Design review of the part shown in the three views and the two pictorial views. Dimensions are in mm from the part's minimum x, y and z. Give positions to 0.01 mm unless a question says otherwise; leave off trailing zeros. Order: outer loops, then holes, each group sorted by start corner. A loop starts at its lowest first (then second) coordinate and runs counter-clockwise, first axis right, second up.
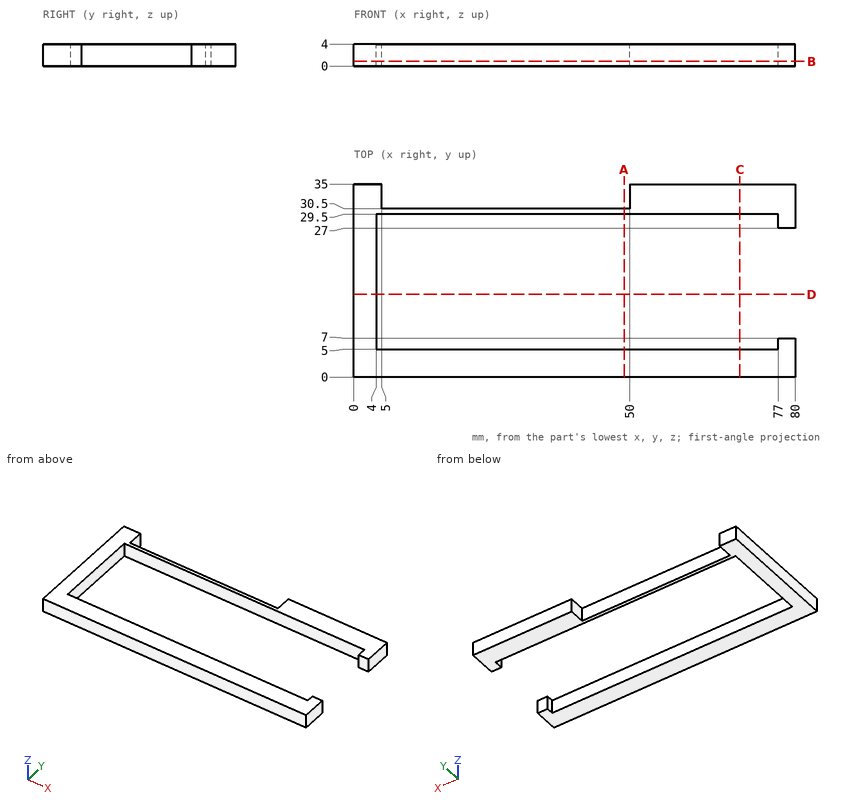
1) We need section A-A on x = 49. Give the boundary of the cut face in (y, z), then the cut area to 3 significant figures.
Answer sheet:
outline: (0, 0) - (5, 0) - (5, 4) - (0, 4) - close; (29.5, 0) - (30.5, 0) - (30.5, 4) - (29.5, 4) - close
area: 24.0 mm2
2) To check wall thickness, follow line 1 (Y direction, x = 39, z = 0.3); line 2 (Y direction, x = 51, z = 2.45); line 3 (X direction, y = 6, z = 3.2). State the ranges of each line that lie inside material, in increasing order.
Answer sheet:
line 1: y = 0 to 5, 29.5 to 30.5
line 2: y = 0 to 5, 29.5 to 35
line 3: x = 0 to 4, 77 to 80
3) Clearance check with flat-ended pins moving along their axes: pin 1 (1.2 mm diameter, centred on y = 20, z = 2.5, fed in from +X); pin 2 (1.2 mm diameter, centred on x = 30, z = 1.5, fed in from +Y). State where each tip first meets the part, or that it passes through.
Answer sheet:
pin 1: stops at x = 4
pin 2: stops at y = 30.5
4) We need section D-D on y = 15. Give the boundary of the cut face in (x, z), then the cut area to 3 significant figures.
Answer sheet:
outline: (0, 0) - (4, 0) - (4, 4) - (0, 4) - close
area: 16.0 mm2
5) We need section C-C on x = 70. Give the boundary of the cut face in (y, z), then the cut area to 3 significant figures.
Answer sheet:
outline: (0, 0) - (5, 0) - (5, 4) - (0, 4) - close; (29.5, 0) - (35, 0) - (35, 4) - (29.5, 4) - close
area: 42.0 mm2
6) We need section B-B on z = 0.85. Give the boundary of the cut face in (x, y), then the cut area to 3 significant figures.
Answer sheet:
outline: (0, 0) - (80, 0) - (80, 7) - (77, 7) - (77, 5) - (4, 5) - (4, 29.5) - (77, 29.5) - (77, 27) - (80, 27) - (80, 35) - (50, 35) - (50, 30.5) - (5, 30.5) - (5, 35) - (0, 35) - close
area: 749 mm2
